Geometry check sheet. Reference: the model listing, model coordinates, mm. A direction names the side the tool comes from. Coordinates: 2 decimals unless noted, no trailing zeros. Loops run counter-clockwise (first coordinate to the right, second up) from the corner with the lowest first, then second, coordinate; pieces in that order, holes last.
from build123d import *

# Parameters (mm, degrees)
EXTRUDE_1_DEPTH          = 70
CUT_EXTRUDE_1_DEPTH      = 3
CUT_EXTRUDE_1_DEPTH_BACK = 79.421935707
SKETCH_2_R               = 1.5
SKETCH_6_R               = 2.7
SKETCH_6_R_2             = 1.5
CUT_EXTRUDE_3_DEPTH      = 21.2
SKETCH_7_W               = 40
SKETCH_7_H               = 5.8
EXTRUDE_2_DEPTH          = 70
CUT_EXTRUDE_4_REACH      = 96.868
SKETCH_8_R               = 2.5


with BuildPart() as part:
    # 草图1 → 凸台-拉伸1 (new body)
    with BuildSketch(Plane(origin=(0, 0, 0), x_dir=(1, 0, 0), z_dir=(0, 1, 0))):
        with BuildLine():
            Line((0, 25), (0, 19.2))
            ThreePointArc((0, 19.2), (-19.2, 0), (0, -19.2))
            Line((0, -19.2), (0, -25))
            ThreePointArc((0, -25), (-25, 0), (0, 25))
        make_face()
    extrude(amount=EXTRUDE_1_DEPTH)

    # 草图2 → 切除-拉伸1 (cut, two sides: drawn at the far end of the back side and taken through both)
    with BuildSketch(Plane(origin=(0, 0, 0), x_dir=(0, 0, -1), z_dir=(1, 0, 0)).offset(-CUT_EXTRUDE_1_DEPTH_BACK)):
        with Locations(Location((0, 58.75, 0), (0, 0, 180))):
            Circle(SKETCH_2_R)
        with Locations(Location((0, 44.75, 0), (0, 0, 180))):
            Circle(SKETCH_2_R)
        with Locations(Location((0, 24, 0), (0, 0, 180))):
            Circle(SKETCH_2_R)
        with Locations(Location((0, 10, 0), (0, 0, 180))):
            Circle(SKETCH_2_R)
    extrude(amount=CUT_EXTRUDE_1_DEPTH + CUT_EXTRUDE_1_DEPTH_BACK, mode=Mode.SUBTRACT)

    # 草图6 → 切除-拉伸3 (cut)
    # profile 1 of 4: a face of its own
    with BuildSketch(Plane(origin=(0, 0, 0), x_dir=(0, 0, -1), z_dir=(1, 0, 0))):
        with Locations((0, 58.75)):
            Circle(SKETCH_6_R)
        with Locations(Location((0, 58.75, 0), (0, 0, 180))):
            Circle(SKETCH_6_R_2, mode=Mode.SUBTRACT)
    # profile 2 of 4: a face of its own
    with BuildSketch(Plane(origin=(0, 0, 0), x_dir=(0, 0, -1), z_dir=(1, 0, 0))):
        with Locations((0, 44.75)):
            Circle(SKETCH_6_R)
        with Locations(Location((0, 44.75, 0), (0, 0, 180))):
            Circle(SKETCH_6_R_2, mode=Mode.SUBTRACT)
    # profile 3 of 4: a face of its own
    with BuildSketch(Plane(origin=(0, 0, 0), x_dir=(0, 0, -1), z_dir=(1, 0, 0))):
        with Locations((0, 24)):
            Circle(SKETCH_6_R)
        with Locations(Location((0, 24, 0), (0, 0, 180))):
            Circle(SKETCH_6_R_2, mode=Mode.SUBTRACT)
    # profile 4 of 4: a face of its own
    with BuildSketch(Plane(origin=(0, 0, 0), x_dir=(0, 0, -1), z_dir=(1, 0, 0))):
        with Locations((0, 10)):
            Circle(SKETCH_6_R)
        with Locations(Location((0, 10, 0), (0, 0, 180))):
            Circle(SKETCH_6_R_2, mode=Mode.SUBTRACT)
    extrude(amount=-CUT_EXTRUDE_3_DEPTH, mode=Mode.SUBTRACT)

    # 草图7 → 凸台-拉伸2 (add)
    with BuildSketch(Plane(origin=(0, 70, 0), x_dir=(1, 0, 0), z_dir=(0, 1, 0))):
        with Locations((20, 22.1)):
            Rectangle(SKETCH_7_W, SKETCH_7_H)
        with Locations((20, -22.1)):
            Rectangle(SKETCH_7_W, SKETCH_7_H)
    extrude(amount=-EXTRUDE_2_DEPTH)

    # 切除-拉伸4: up to this face of the body (flat: up to its plane)
    cut_extrude_4_end = Plane(part.part.faces().sort_by_distance((20, 35, -25))[0])
    # 草图8 → 切除-拉伸4 (cut, up to the picked face)
    with BuildSketch(Plane.XY.offset(25), mode=Mode.PRIVATE) as cut_extrude_4_sk1:
        with Locations((21.8, 45)):
            Circle(SKETCH_8_R)
    cut_extrude_4_tool1 = split(extrude(cut_extrude_4_sk1.sketch, amount=-CUT_EXTRUDE_4_REACH, mode=Mode.PRIVATE), bisect_by=cut_extrude_4_end, keep=Keep.BOTH, mode=Mode.PRIVATE)
    add(cut_extrude_4_tool1.solids().sort_by(Axis((21.8, 45, 25), (0, 0, -1)))[0], mode=Mode.SUBTRACT)


solid = part.part
1) Section check C-C on y = 36. Record the cut outline in (x, z).
Data:
outline: (0, -25) - (40, -25) - (40, -19.2) - (0, -19.2) arc R19.2 cw to (0, 19.2) - (40, 19.2) - (40, 25) - (0, 25) arc R25 ccw to start
2) Material ranges on probe 1 along Y at (x, z) = (-24, 0); probe 2 along Y at (x, z) = (-20.4, 0); probe 3 along Z at (x, y) = (10, 9), recorded low to high.
Data:
probe 1: y = 0 to 8.5, 11.5 to 22.5, 25.5 to 43.25, 46.25 to 57.25, 60.25 to 70
probe 2: y = 0 to 7.3, 12.7 to 21.3, 26.7 to 42.05, 47.45 to 56.05, 61.45 to 70
probe 3: z = -25 to -19.2, 19.2 to 25
3) Section check A-A on x = 14. Record the cut outline in (y, z), and give its area (3 significant figures).
Data:
outline: (0, -25) - (70, -25) - (70, -19.2) - (0, -19.2) - close; (0, 19.2) - (70, 19.2) - (70, 25) - (0, 25) - close
area: 812 mm2
4) Access from +Z, -Z, +X, -X, +Y, -Y to the whole of each face (thin tool, end or side, straight path). Record for faces 1 (the flat face through (20, 35, 19.2)), 2 (the flat face through (-21.2, 57.6, -1.2)), 3 (the flat face through (-5, 70, -19)).
Data:
face 1: +X, +Y, -Y
face 2: +X
face 3: +Z, -Z, +X, -X, +Y
5) Section check D-D on z = 0. Count the separate pieces of the cut face and the enclosed holes in it, and give its area (3 significant figures).
Data:
separate pieces: 5
enclosed holes: 0
area: 317 mm2
6) Section check B-B on y = 58.75. Record the cut outline in (x, z).
Data:
outline: (-24.95, -1.5) arc R25 ccw to (0, -25) - (40, -25) - (40, -19.2) - (0, -19.2) arc R19.2 cw to (-19.01, -2.7) - (-21.2, -2.7) - (-21.2, -1.5) - close; (-24.95, 1.5) - (-21.2, 1.5) - (-21.2, 2.7) - (-19.01, 2.7) arc R19.2 cw to (0, 19.2) - (40, 19.2) - (40, 25) - (0, 25) arc R25 ccw to start
7) Mould release check, pull along X, two halves, no side actions. Record for faces 4 (the cylindrical face through (-19.195, 34.51, -0.422)), 5 (the cylindrical face through (-24.994, 34.51, 0.55)), 6 (the cylindrical face through (21.26, 42.56, -22.06)), 7 (the flat face through (20, 35, -19.2)): +X half, -X half, draft (parallel to the pull), parting line (faces both ways), or undercut.
Data:
face 4: +X half
face 5: -X half
face 6: undercut
face 7: draft
8) Depth check by flat-ended pin: pin 1 (5 mm diameter, centred on y = 24, z = 0, fed in from +X); pin 2 (3 mm diameter, centred on y = 47.5, z = -7.5, fed in from +X); pin 3 (8.5 mm diameter, centred on y = 44.75, z = 0, fed in from +X). Enter the tip coordinate at first touch or a pass-through.
Data:
pin 1: stops at x = -21.2
pin 2: stops at x = -16.96
pin 3: stops at x = -18.72
